```python
from build123d import *

# Parameters (mm, degrees)
F0_R      = 7.1015967563
F1_DEPTH  = 12.7
F2_R      = 5.6788395521
F3_DEPTH  = 19.05
F4_R      = 4.6676560737
F5_DEPTH  = 13.97
F6_R      = 2.5243045871
F7_DEPTH  = 5.08
F8_R      = 2.6650653171
F9_DEPTH  = 43.18
F10_R     = 0.7037770969
F11_DEPTH = 25.4
F12_SIZE  = 0.381


# Not quite as in the source:
# - the program builds the solid bodies; features that only make, move or delete a surface that nothing else refers to are left out


with BuildPart() as f1:
    # F0 (on Right) → F1 (new body)
    with BuildSketch(Plane.YZ):
        Circle(F0_R)
    extrude(amount=F1_DEPTH)

    # F2 (on face) → F3 (join)
    with BuildSketch(Plane.YZ.offset(12.7)):
        Circle(F2_R)
    extrude(amount=F3_DEPTH)

    # F4 (on face) → F5 (join)
    with BuildSketch(Plane(origin=(0, 0, 0), x_dir=(0, -1, 0), z_dir=(-1, 0, 0))):
        Circle(F4_R)
    extrude(amount=F5_DEPTH)

    # F6 (on face) → F7 (join)
    with BuildSketch(Plane(origin=(-13.97, 0, 0), x_dir=(0, -1, 0), z_dir=(-1, 0, 0))):
        Circle(F6_R)
    extrude(amount=F7_DEPTH)

    # F8 (on face) → F9 (cut)
    with BuildSketch(Plane.YZ.offset(31.75)):
        Circle(F8_R)
    extrude(amount=-F9_DEPTH, mode=Mode.SUBTRACT)

    # F10 (on face) → F11 (cut)
    with BuildSketch(Plane(origin=(-19.05, 0, 0), x_dir=(0, -1, 0), z_dir=(-1, 0, 0))):
        Circle(F10_R)
    extrude(amount=-F11_DEPTH, mode=Mode.SUBTRACT)

    # F12
    f12_edges = [f1.edges().sort_by_distance(p)[0] for p in [
        (-11.43, 0.703777, 0),
    ]]
    chamfer(f12_edges, length=F12_SIZE)


solid = f1.part
```
Part model, mm, in its own coordinate system. A direction names the side the tool comes from. Round coordinates to 2 decimals unless told otherwise and drop trailing zeros. Loops run counter-clockwise (first coordinate to the right, second up) from the corner with the lowest first, then second, coordinate; pieces in that order, holes last.
1. Slice it at C-C (x = 22.5). Give the cut face in (y, z), and give its area (3 significant figures).
Solutions:
outline: circle Ø11.36 at (0, 0); hole circle Ø5.33 at (0, 0)
area: 79.0 mm2
2. Slice it at D-D (z = 3.75). Give the cut face in (x, y), and give its area (3 significant figures).
Solutions:
outline: (-13.97, -2.78) - (0, -2.78) - (0, -6.03) - (12.7, -6.03) - (12.7, -4.26) - (31.75, -4.26) - (31.75, 4.26) - (12.7, 4.26) - (12.7, 6.03) - (0, 6.03) - (0, 2.78) - (-13.97, 2.78) - close
area: 393 mm2
3. Drill centre lines: line 1 along Z through (x, y) = (18, 0); line 2 along Z through (x, y) = (12, 0); line 3 along X through (y, z) = (-0.75, -2.5). Where is each one in solid material? Low to high.
Solutions:
line 1: z = -5.68 to -2.67, 2.67 to 5.68
line 2: z = -7.1 to -2.67, 2.67 to 7.1
line 3: x = -13.97 to -11.43
4. Slice it at A-A (y = 0). Give the cut face in (x, z), and give its area (3 significant figures).
Solutions:
outline: (-19.05, -2.52) - (-13.97, -2.52) - (-13.97, -4.67) - (0, -4.67) - (0, -7.1) - (12.7, -7.1) - (12.7, -5.68) - (31.75, -5.68) - (31.75, -2.67) - (-11.43, -2.67) - (-11.43, -1.08) - (-11.81, -0.7) - (-19.05, -0.7) - close; (-19.05, 0.7) - (-11.81, 0.7) - (-11.43, 1.08) - (-11.43, 2.67) - (31.75, 2.67) - (31.75, 5.68) - (12.7, 5.68) - (12.7, 7.1) - (0, 7.1) - (0, 4.67) - (-13.97, 4.67) - (-13.97, 2.52) - (-19.05, 2.52) - close
area: 312 mm2
5. Flat gauge pins, fed straight in: pin 1 (5 mm diameter, centred on x = -7.5, z = 2.5, fed in from -Y); pin 2 (2 mm diameter, centred on x = 25.5, y = -1.5, fed in from -Z); pin 3 (1 mm diameter, centred on x = -13, y = 4, fed in from +Z). Where does each tip first touch, or does it go through?
Solutions:
pin 1: stops at y = -4.67
pin 2: stops at z = -5.66
pin 3: stops at z = 3.09
6. Two-plate mould, pull along Y, no slides. Class faces 1 (the face through (-11.43, 1, -1)), 2 (the face through (31.75, -3, -1)), 3 (the face through (-6.887, -2.154, -4.141)): pulls with the +Y half, pulls with the -Y half, needs draft (parallel to the pull), parting line crosses it, or undercut.
Solutions:
face 1: undercut
face 2: needs draft
face 3: parting line crosses it
7. 3-axis set-ups, long thin cutter, end or side, ignore diameter. For faces 4 (the face through (-15.481, 0.703, 0.031)), 5 (the face through (-13.97, -2, -2)), 6 (the face through (12.7, -5, -3)): which of +Z, -Z, +X, -X, +Y, -Y reach the whole face in a straight line?
Solutions:
face 4: +X, -X
face 5: -X
face 6: +X
